```python
from build123d import *

# Parameters (mm, degrees)
SKETCH1_W               = 22.6822
SKETCH1_H               = 22.6822
SKETCH1_W_2             = 20.1422
SKETCH1_H_2             = 20.1422
BOSS_EXTRUDE1_DEPTH     = 1303.02
FILLET1_R               = 2.54
F_1_4_CLEARANCE_HOLE1_D = 6.7564


with BuildPart() as part:
    # Sketch1 → Boss-Extrude1 (new body)
    with BuildSketch(Plane(origin=(0, 0, 0), x_dir=(1, 0, 0), z_dir=(0, 1, 0))):
        Rectangle(SKETCH1_W, SKETCH1_H)
        Rectangle(SKETCH1_W_2, SKETCH1_H_2, mode=Mode.SUBTRACT)
    extrude(amount=BOSS_EXTRUDE1_DEPTH)

    # Fillet1
    fillet1_edges = [part.edges().sort_by_distance(p)[0] for p in [
        (10.0711, 651.51, 10.0711),
        (10.0711, 651.51, -10.0711),
        (-10.0711, 651.51, -10.0711),
        (-10.0711, 651.51, 10.0711),
        (11.3411, 651.51, 11.3411),
        (-11.3411, 651.51, 11.3411),
        (-11.3411, 651.51, -11.3411),
        (11.3411, 651.51, -11.3411),
    ]]
    fillet(fillet1_edges, radius=FILLET1_R)

    # 1/4 Clearance Hole1 (through all)
    with Locations(Plane(origin=(11.3411, 0, 0), x_dir=(0, 0, -1), z_dir=(1, 0, 0))):
        with Locations((0, 1287.145)):
            Hole(F_1_4_CLEARANCE_HOLE1_D / 2)


solid = part.part
```
Model file for the job. Use its own axes, mm. Give positions to 0.01 mm unless a question says otherwise; leave off trailing zeros. Write each loop counter-clockwise with the first axis right and the second up, starting at its lowest first coordinate (ties: lowest second). Pieces come first, ordered by that corner, then holes. Notation, with made-up numbers: M -1.5,46.5 L 16.5,46.5 A21 ccw 16.5,62.5 Z; hole C 8,63 d2. An arc over 180 degrees is marked long. Use a Markdown table: item, result.
1) Cut at B-B (y = 644). List the corners of the cut face in (x, z).
Responses:
| item | result |
|---|---|
| outline | M -11.34,-8.8 A2.54 ccw -8.8,-11.34 L 8.8,-11.34 A2.54 ccw 11.34,-8.8 L 11.34,8.8 A2.54 ccw 8.8,11.34 L -8.8,11.34 A2.54 ccw -11.34,8.8 Z; hole M -10.07,-7.53 A2.54 ccw -7.53,-10.07 L 7.53,-10.07 A2.54 ccw 10.07,-7.53 L 10.07,7.53 A2.54 ccw 7.53,10.07 L -7.53,10.07 A2.54 ccw -10.07,7.53 Z |
2) Drill centre lines: line 1 (Y direction, x = 10.8, z = 0); line 2 (X direction, y = 763, z = 2.75). Where is each one in solid material? Low to high. Write a range as from..to.
Responses:
| item | result |
|---|---|
| line 1 | y = 0..1283.77, 1290.52..1303.02 |
| line 2 | x = -11.34..-10.07, 10.07..11.34 |
3) Cut at A-A (x = -1.5). List the corners of the cut face in (y, z), and give its area (3 significant figures).
Responses:
| item | result |
|---|---|
| outline | M 0,-11.34 L 1303.02,-11.34 L 1303.02,-10.07 L 0,-10.07 Z; M 0,10.07 L 1303.02,10.07 L 1303.02,11.34 L 0,11.34 Z |
| area | 3,310 mm2 |
